CAD build for the part. Positions are in the model's coordinates, mm. Face numbers are marked on the shaded views. Give positions to 0.01 mm unless a question says otherwise; leave off trailing zeros. Loops run counter-clockwise (first coordinate to the right, second up) from the corner with the lowest first, then second, coordinate; pieces in that order, holes last.
Item 1: Mould opens along X. For the marked faces 1, 2, 3 and 4 say: released by +X, released by -X, zero draft, split by the parting line, or undercut.
Item 2: Probe probe 1 along Z at (x, y) = (1, -2.5); probe 2 along Z at (x, y) = (-8.5, 1.5); probe 3 along Y at (x, z) = (38, 26.5). List the from-to ranges inside material, lowest first.
Item 3: Drop flat-ended pins along their axis: P1, Ø10, axis at x = 46, y = 4.5, coming from the +Z side; P2, Ø8, axis at x = 43.5, y = 2.5, coming from the -Z side; P3, Ø6, axis at x = 13.5, y = -1.5, coming from the -Z side. Give the stop position or say it passes through.
Item 4: Saw through at A-A on y = 1. Give the cut face in (x, z).
Item 5: Saw through at C-C on z = 18.5. Give the cut face in (x, y), plus the area to 3 significant figures.
Item 6: Saw through at D-D on x = 27. Give the cut face in (y, z).
Item 7: Saw through at B-B on z = 24.5. Give the cut face in (x, y).
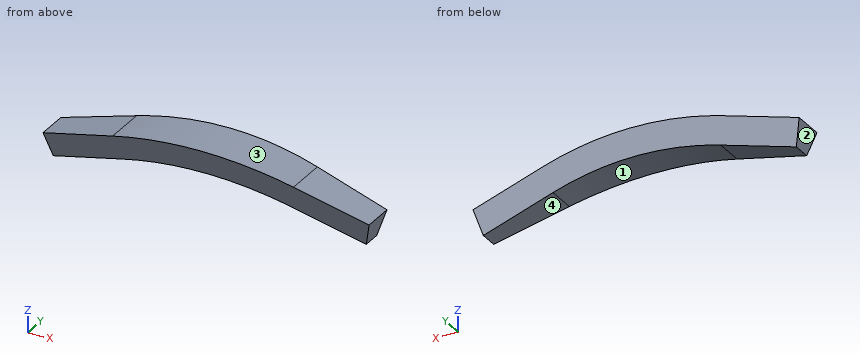
from build123d import *

# Parameters (mm, degrees)
F1_DEPTH = 15
F3_DEPTH = 100
F5_DEPTH = 25


with BuildPart() as f1:
    # F0 (on Front) → F1 (new body, symmetric)
    with BuildSketch(Plane.XZ):
        with BuildLine():
            ThreePointArc((-32.9082667369, 19.25967), (0, 23.6280366002), (32.9082667369, 19.25967))
            Line((32.9082667369, 19.25967), (61.8693159107, 11.43296))
            Line((61.8693159107, 11.43296), (65, 23.01738))
            Line((65, 23.01738), (36.0389508262, 30.84409))
            ThreePointArc((36.0389508262, 30.84409), (0, 35.6280353337), (-36.0389508262, 30.84409))
            Line((-36.0389508262, 30.84409), (-65, 23.01738))
            Line((-65, 23.01738), (-61.8693159107, 11.43296))
            Line((-61.8693159107, 11.43296), (-32.9082667369, 19.25967))
        make_face()
    extrude(amount=F1_DEPTH, both=True)

    # F2 (on Right) → F3 (cut, symmetric)
    with BuildSketch(Plane.YZ):
        Polygon((-1.875644347, 7), (-17, 63.4448637287), (-17, 0), (0, 0), (17, 0), (17, 63.4448637287), (1.875644347, 7), align=None)
    extrude(amount=F3_DEPTH, both=True, mode=Mode.SUBTRACT)

    # F4 (on Front) → F5 (cut, symmetric)
    with BuildSketch(Plane.XZ):
        with BuildLine():
            Line((62.3910966473, 13.3636968704), (33.4300474735, 21.1904068704))
            ThreePointArc((33.4300474735, 21.1904068704), (0, 25.6280366002), (-33.4300474735, 21.1904068704))
            Line((-33.4300474735, 21.1904068704), (-62.3910966473, 13.3636968704))
            Line((-62.3910966473, 13.3636968704), (-61.8693159107, 11.43296))
            Line((-61.8693159107, 11.43296), (-32.9082667369, 19.25967))
            ThreePointArc((-32.9082667369, 19.25967), (0, 23.6280366002), (32.9082667369, 19.25967))
            Line((32.9082667369, 19.25967), (61.8693159107, 11.43296))
            Line((61.8693159107, 11.43296), (62.3910966473, 13.3636968704))
        make_face()
    extrude(amount=F5_DEPTH, both=True, mode=Mode.SUBTRACT)


solid = f1.part
Results below:
1. face 1: undercut
1. face 2: released by -X
1. face 3: split by the parting line
1. face 4: undercut
2. probe 1: z = 25.62 to 35.62
2. probe 2: z = 25.35 to 35.37
2. probe 3: y = -7.1 to 7.1
3. P1: stops at z = 29.5
3. P2: stops at z = 17.39
3. P3: stops at z = 24.56
4. outline: (-65, 23.02) - (-62.39, 13.36) - (-33.43, 21.19) arc R128.14 cw to (33.43, 21.19) - (62.39, 13.36) - (65, 23.02) - (36.04, 30.84) arc R138.14 ccw to (-36.04, 30.84) - close
5. outline: (-63.78, -4.96) - (-43.39, -4.96) - (-43.39, 4.96) - (-63.78, 4.96) - close; (43.39, -4.96) - (63.78, -4.96) - (63.78, 4.96) - (43.39, 4.96) - close
5. area: 404 mm2
6. outline: (-8.83, 32.96) - (-6.1, 22.75) - (6.1, 22.75) - (8.83, 32.96) - close
7. outline: (-59.51, -6.56) - (-16.97, -6.56) - (-16.97, 6.56) - (-59.51, 6.56) - close; (16.97, -6.56) - (59.51, -6.56) - (59.51, 6.56) - (16.97, 6.56) - close
